```python
from build123d import *

# Parameters (mm, degrees)
F1_DEPTH  = 25.4
F2_R      = 12.7
F3_DEPTH  = 25.4
F4_R      = 12.7
F5_DEPTH  = 25.4
F6_DEPTH  = 25.4
F8_DEPTH  = 33.02
F9_R      = 6.35
F10_DEPTH = 5.08


with BuildPart() as f1:
    # F0 (on Top) → F1 (new body)
    with BuildSketch(Plane.XY):
        with BuildLine():
            Line((13.423362, -72.093714), (38.1, 0))
            ThreePointArc((38.1, 0), (0, 38.1), (-38.1, 0))
            Line((-38.1, 0), (-13.423362, -72.093714))
            Line((-13.423362, -72.093714), (-12.7, -72.093714))
            Line((-12.7, -72.093714), (-12.622174, -72.093714))
            ThreePointArc((-12.622174, -72.093714), (0, -86.197534), (12.622174, -72.093714))
            Line((12.622174, -72.093714), (12.7, -72.093714))
            Line((12.7, -72.093714), (13.423362, -72.093714))
        make_face()
    extrude(amount=F1_DEPTH)

    # F2 (on face) → F3 (cut)
    with BuildSketch(Plane.XY.offset(25.4)):
        with Locations((0, 22.86)):
            Circle(F2_R)
    extrude(amount=-F3_DEPTH, mode=Mode.SUBTRACT)

    # F4 (on face) → F5 (cut)
    with BuildSketch(Plane.XY.offset(25.4)):
        with Locations((-21.741152, 7.064128)):
            Circle(F4_R)
    extrude(amount=-F5_DEPTH, mode=Mode.SUBTRACT)

    # F4 (on face) → F6 (cut)
    with BuildSketch(Plane.XY.offset(25.4)):
        with Locations((0, 22.86)):
            Circle(F4_R)
        with Locations((-21.741152, 7.064128)):
            Circle(F4_R)
        with Locations((-13.436771, -18.494128)):
            Circle(F4_R)
        with Locations((13.436771, -18.494128)):
            Circle(F4_R)
        with Locations((21.741152, 7.064128)):
            Circle(F4_R)
    extrude(amount=-F6_DEPTH, mode=Mode.SUBTRACT)

    # F7 (on Top) → F8 (join)
    with BuildSketch(Plane.XY):
        with BuildLine():
            Line((-7.010239, -0.563764), (-7.010239, -62.219993))
            ThreePointArc((-7.010239, -62.219993), (0.533631, -85.363339), (6.098, -61.666034))
            Line((6.098, -61.666034), (7.001797, -0.570687))
            ThreePointArc((7.001797, -0.570687), (0.005459, 19.025547), (-7.010239, -0.563764))
        make_face()
    extrude(amount=F8_DEPTH)

    # F9 (on face) → F10 (join)
    with BuildSketch(Plane.XY.offset(33.02)):
        with Locations((0, 7.976549)):
            Circle(F9_R)
        with Locations((0, -72.736099)):
            Circle(F9_R)
    extrude(amount=F10_DEPTH)


solid = f1.part
```
Can you work these out from the model? Positions are in its coordinate system, mm. A direction names the side the tool comes from. Give positions to 0.01 mm unless a question says otherwise; leave off trailing zeros. Order: outer loops, then holes, each group sorted by start corner. A loop starts at its lowest first (then second) coordinate and runs counter-clockwise, first axis right, second up. Notation, with made-up numbers: M -24,48.5 L 15,48.5 A29 ccw 15,70.5 Z; hole C 60,-8.5 d6. An arc over 180 degrees is marked long. One line per item, written item: value.
1) I want a section at C-C, the plane y = -23.5. List the corners of the cut face in (x, z) for me.
Answer sheet:
outline: M -30.06,0 L -25.11,0 L -25.11,25.4 L -30.06,25.4 Z; M -7.01,0 L 6.66,0 L 6.66,33.02 L -7.01,33.02 Z; M 25.11,0 L 30.06,0 L 30.06,25.4 L 25.11,25.4 Z
2) For P1, Ø10, axis at y = -55, z = 9, coming from the +X side; P2, Ø23, axis at x = 21.74, y = 7.06, coming from the +Z side; P3, Ø2, axis at y = -32.5, z = 5, coming from the +X side, each with a flat end and sliding along its axis, tell me the tip position at first contact or that it passes through.
Answer sheet:
P1: stops at x = 20.99
P2: stops at z = 33.02
P3: stops at x = 27.32
3) Please list where these lines run through material, in increasing order: line 1 along X through (y, z) = (-1.5, 3); line 2 along Y through (x, z) = (0, 5); line 3 along Y through (x, z) = (7.5, 3).
Answer sheet:
line 1: x = -37.59 to -31.12, -12.36 to 12.36, 31.12 to 37.59
line 2: y = -86.2 to 19.03, 35.56 to 38.1
line 3: y = -83.75 to -29.72, -7.27 to 16.09, 33.11 to 37.35
4) On a 3-axis mill with a long thin cutter (end or side, diameter ignored), from which of +Z, -Z, +X, -X, +Y, -Y can I reach the whole of each face in a straight line? I mean faces 4 (the face through (0, -32, 33.02)), 5 (the face through (-1, -23, 0)). Say none if no direction works.
Answer sheet:
face 4: +Z
face 5: -Z, +X, -X, +Y, -Y
5) I want a section at B-B, the plane x = 0. List the corners of the cut face in (y, z) for me.
Answer sheet:
outline: M -86.2,0 L 19.03,0 L 19.03,33.02 L 14.33,33.02 L 14.33,38.1 L 1.63,38.1 L 1.63,33.02 L -66.39,33.02 L -66.39,38.1 L -79.09,38.1 L -79.09,33.02 L -85.37,33.02 L -85.37,25.4 L -86.2,25.4 Z; M 35.56,0 L 38.1,0 L 38.1,25.4 L 35.56,25.4 Z
6) I want a section at A-A, the plane y = 22.86. List the corners of the cut face in (x, z) for me, plus the area to 3 significant figures.
Answer sheet:
outline: M -30.48,0 L -12.7,0 L -12.7,25.4 L -30.48,25.4 Z; M 12.7,0 L 30.48,0 L 30.48,25.4 L 12.7,25.4 Z
area: 903 mm^2
7) I want a section at D-D, the plane z = 2.5. Count the separate pieces of the cut face and the enclosed holes in it, plus the area to 3 significant figures.
Answer sheet:
separate pieces: 1
enclosed holes: 5
area: 4,080 mm^2
8) We'd pull the mould along X, two halves only. Please class faces 1 (the face through (34.4, 6.04, 12.88)), 2 (the face through (-25.934, -35.542, 12.522)), 3 (the face through (0.84, 38.09, 12.52)): released by +X, released by -X, zero draft, split by the parting line, or undercut.
Answer sheet:
face 1: undercut
face 2: released by -X
face 3: split by the parting line
